Can you work these out from the model? Positions are in its coordinate system, mm. A direction names the side the tool comes from. Coordinates: 2 decimals unless noted, no trailing zeros. Order: outer loops, then holes, each group sorted by start corner. A loop starts at its lowest first (then second) coordinate and runs counter-clockwise, first axis right, second up. Notation, with made-up numbers: (-8, -37.75) -> (-1, -37.75) arc R26 cw to (-1, -1.75) -> close; hole circle Ø4 at (-1, 9). An arc over 180 degrees is marked (long way). Use a Markdown table: item, result. Add a question column.
1. For faces 4 (the flat face through (1.724, 2.913, 1.014)), 5 (the cylindrical face through (-0.867, 1.873, 3.905)), 6 (the flat face through (2, 0, -2)), which set-ups out of +Z, -Z, +X, -X, +Y, -Y let a thin tool reach every point of the face, with its end or its side?
2. If I drill on line 1 along Y through (x, z) = (-0.25, 1); line 2 along Y through (x, z) = (1, -3); line 3 along X through (y, z) = (-16.25, -1.5), over which ranges is the centre line in solid material (lowest first)? Write a range as from..to.
3. Suppose I cut it at A-A, the plane x = 0. List the corners of the cut face in (y, z) for me.
4. Suppose I cut it at B-B, the plane y = -20. List the corners of the cut face in (x, z) for me.
5. For pin 1 Ø3 at (x, y) = (-2.5, -21) entering from +Z; pin 2 Ø1.5 at (x, y) = (1.5, -3.5) entering from +Z; pin 3 Ø1.5 at (x, y) = (3, -20) entering from +Z, each with a flat end and sliding along its axis, tell me the tip position at first contact or that it passes through.
6. We'd pull the mould along X, two halves only. Please class faces 1 (the cylindrical face through (-0.54, -12.18, -2.44)), 2 (the flat face through (0, -25, 0)), 3 (the flat face through (-1.724, 2.913, -1.014)): pulls with the +X half, pulls with the -X half, needs draft (parallel to the pull), parting line crosses it, or undercut.
```python
from build123d import *

# Parameters (mm, degrees)
SKETCH_1_R          = 4
EXTRUDE_1_DEPTH     = 4
SKETCH_2_R          = 2.5
EXTRUDE_2_DEPTH     = 25
CUT_EXTRUDE_1_DEPTH = 2
CHAMFER_1_SIZE      = 0.2
CHAMFER_2_SIZE      = 0.3


with BuildPart() as part:
    # 草图1 → 凸台-拉伸1 (new body)
    with BuildSketch(Plane(origin=(0, 0, 0), x_dir=(1, 0, 0), z_dir=(0, 1, 0))):
        Circle(SKETCH_1_R)
    extrude(amount=EXTRUDE_1_DEPTH)

    # 草图2 → 凸台-拉伸2 (add)
    with BuildSketch(Plane.XZ):
        Circle(SKETCH_2_R)
    extrude(amount=EXTRUDE_2_DEPTH)

    # 草图11 → 切除-拉伸1 (cut)
    with BuildSketch(Plane(origin=(0, 4, 0), x_dir=(1, 0, 0), z_dir=(0, 1, 0))):
        Polygon((1.154954177, 1.999853541), (-1.154446882, 2.000146427), (-2.309401058, 0.000292887), (-1.154954177, -1.999853541), (1.154446882, -2.000146427), (2.309401058, -0.000292887), align=None)
    extrude(amount=-CUT_EXTRUDE_1_DEPTH, mode=Mode.SUBTRACT)

    # 倒角1
    chamfer_1_edges = [part.edges().sort_by_distance(p)[0] for p in [
        (1.732177617, 4, -0.999780327),
        (0.000253647, 4, -1.999999984),
        (-1.73192397, 4, -1.000219657),
        (-1.732177617, 4, 0.999780327),
        (-0.000253647, 4, 1.999999984),
        (1.73192397, 4, 1.000219657),
        (-4, 4, 0),
    ]]
    chamfer(chamfer_1_edges, length=CHAMFER_1_SIZE)

    # 倒角2
    chamfer_2_edges = [part.edges().sort_by_distance(p)[0] for p in [
        (-2.5, -25, 0),
    ]]
    chamfer(chamfer_2_edges, length=CHAMFER_2_SIZE)


solid = part.part
```
Worked out:
| question | item | result |
|---|---|---|
| 1 | face 4 | +Y |
| 1 | face 5 | +Y, -Y |
| 1 | face 6 | -Y |
| 2 | line 1 | y = -25..2 |
| 2 | line 2 | y = 0..4 |
| 2 | line 3 | x = -2..2 |
| 3 | outline | (-25, -2.2) -> (-24.7, -2.5) -> (0, -2.5) -> (0, -4) -> (3.8, -4) -> (4, -3.8) -> (4, -2.2) -> (3.8, -2) -> (2, -2) -> (2, 2) -> (3.8, 2) -> (4, 2.2) -> (4, 3.8) -> (3.8, 4) -> (0, 4) -> (0, 2.5) -> (-24.7, 2.5) -> (-25, 2.2) -> close |
| 4 | outline | circle Ø5 at (0, 0) |
| 5 | pin 1 | stops at z = 2.29 |
| 5 | pin 2 | stops at z = 2.38 |
| 5 | pin 3 | stops at z = 1.09 |
| 6 | face 1 | parting line crosses it |
| 6 | face 2 | needs draft |
| 6 | face 3 | undercut |
